```python
from build123d import *

# Parameters (mm, degrees)
SKETCH_1_W          = 53
SKETCH_1_H          = 23
SKETCH_1_R          = 2.5
EXTRUDE_1_DEPTH     = 2
CUT_EXTRUDE_1_DEPTH = 2


with BuildPart() as part:
    # 草图1 → 凸台-拉伸1 (new body)
    with BuildSketch(Plane(origin=(0, 0, 0), x_dir=(1, 0, 0), z_dir=(0, 1, 0))):
        with Locations((26.5, 11.5)):
            Rectangle(SKETCH_1_W, SKETCH_1_H)
        with Locations(Location((28, 11.5, 0), (0, 0, 270))):
            Circle(SKETCH_1_R, mode=Mode.SUBTRACT)
    extrude(amount=EXTRUDE_1_DEPTH)

    # 草图2 → 切除-拉伸1 (cut)
    with BuildSketch(Plane(origin=(0, 2, 0), x_dir=(1, 0, 0), z_dir=(0, 1, 0))):
        Polygon((53, 23), (53, 17), (23, 23), align=None)
        Polygon((23, 0), (53, 6), (53, 0), align=None)
    extrude(amount=-CUT_EXTRUDE_1_DEPTH, mode=Mode.SUBTRACT)


solid = part.part
```
For this review, take the finished solid that the model builds, in its own axes (mm). Round coordinates to 2 decimals unless told otherwise and drop trailing zeros. Write each loop counter-clockwise with the first axis right and the second up, starting at its lowest first coordinate (ties: lowest second). Pieces come first, ordered by that corner, then holes. Notation, with made-up numbers: (-26, -39) -> (23, -39) arc R14 cw to (23, -19) -> close; hole circle Ø6 at (69, 78.25). An arc over 180 degrees is marked (long way). Use one line per item in the form item = value.
1) Take a section at B-B, the plane x = 28. Write out the cut boundary in (y, z), and give its area (3 significant figures).
Found:
outline = (0, -22) -> (2, -22) -> (2, -14) -> (0, -14) -> close; (0, -9) -> (2, -9) -> (2, -1) -> (0, -1) -> close
area = 32.0 mm2
2) Take a section at A-A, the plane z = -11.5. Write out the cut boundary in (x, y), and give its area (3 significant figures).
Found:
outline = (0, 0) -> (25.5, 0) -> (25.5, 2) -> (0, 2) -> close; (30.5, 0) -> (53, 0) -> (53, 2) -> (30.5, 2) -> close
area = 96.0 mm2
3) To check wall thickness, follow L1, parallel to X at y = 1.35, z = -11.5; L2, parallel to X at y = 0.35, z = -10; L3, parallel to Z at x = 47.5, y = 0.6. State the ranges of each line that lie inside material, in increasing order. Write a range as from..to.
Found:
L1 = 0..25.5, 30.5..53
L2 = 0..26, 30..53
L3 = -18.1..-4.9
4) Take a section at C-C, the plane y = 1.05. Write out the cut boundary in (x, z), and give its area (3 significant figures).
Found:
outline = (0, -23) -> (23, -23) -> (53, -17) -> (53, -6) -> (23, 0) -> (0, 0) -> close; hole circle Ø5 at (28, -11.5)
area = 1,020 mm2
5) Mouldability with a two-part tool opening along Z and no side actions: class faces 1 (the flat face through (53, 1, -11)), 2 (the cylindrical face through (30.48, 0.99, -11.83)), 3 (the flat face through (11, 1, -23)) as +Z half, -Z half, draft (parallel to the pull), parting line (faces both ways), or undercut.
Found:
face_1 = draft
face_2 = undercut
face_3 = -Z half
6) Take a section at D-D, the plane x = 36.5. Write out the cut boundary in (y, z).
Found:
outline = (0, -20.3) -> (2, -20.3) -> (2, -2.7) -> (0, -2.7) -> close
7) Clearance check with a flat-ended pin moving along its axis: pin 1 (3 mm diameter, centred on x = 28, z = -11.5, fed in from -Y). State where the tip first meets the part, or that it passes through.
Found:
pin_1 = through
